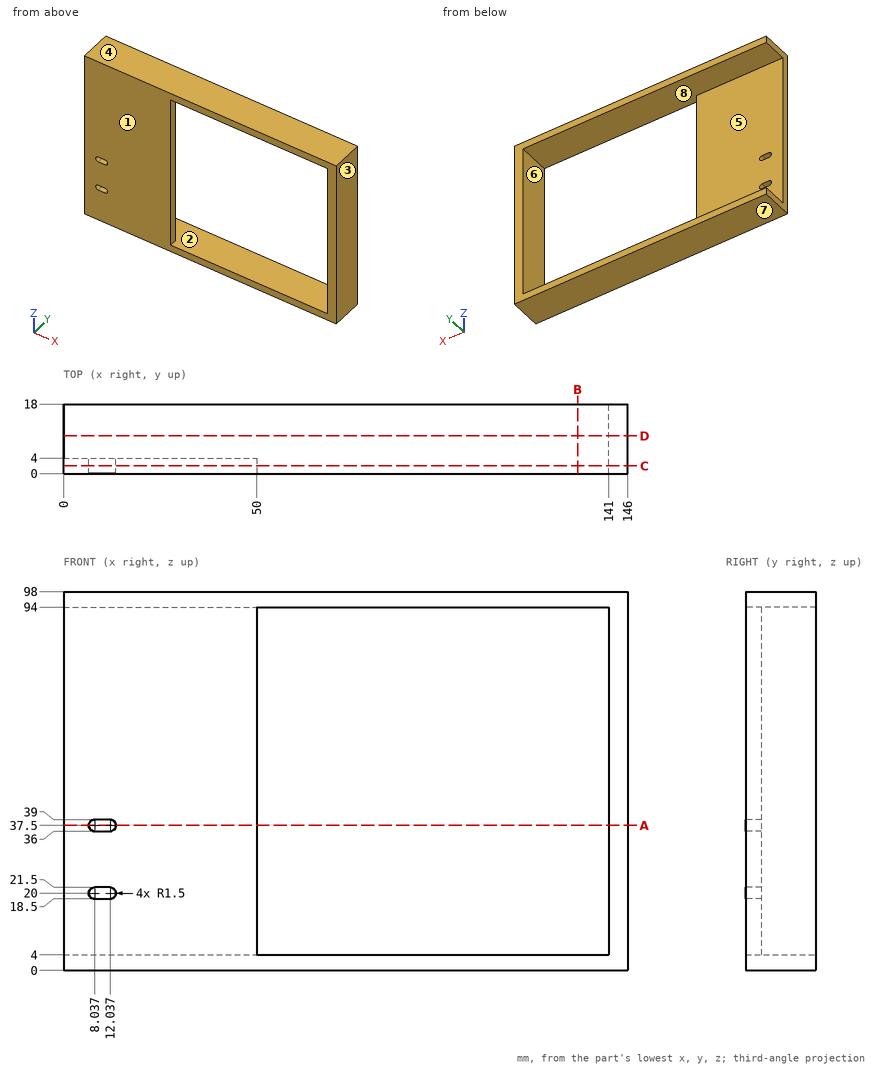
Study the drawing (mm; zero at the part's minimum x, y, z) and answer. A direction names the side the tool comes from. Round coordinates to 2 decimals unless told otherwise and drop trailing zeros. Write each loop counter-clockwise with the first axis right and the second up, starting at its lowest first coordinate (ties: lowest second). Pieces come first, ordered by that corner, then holes.
Q1. Find section A-A on z = 37.5. Determine the outline of the cut face in (x, y).
Values:
outline: (0, 0) - (6.54, 0) - (6.54, 4) - (0, 4) - close; (13.54, 0) - (50, 0) - (50, 4) - (13.54, 4) - close; (141, 0) - (146, 0) - (146, 18) - (141, 18) - close
Q2. Find section C-C on y = 2. Determine the outline of the cut face in (x, z).
Values:
outline: (0, 0) - (146, 0) - (146, 98) - (0, 98) - close; hole (8.04, 18.5) - (12.04, 18.5) arc R1.5 ccw to (12.04, 21.5) - (8.04, 21.5) arc R1.5 ccw to start; hole (8.04, 36) - (12.04, 36) arc R1.5 ccw to (12.04, 39) - (8.04, 39) arc R1.5 ccw to start; hole (50, 4) - (141, 4) - (141, 94) - (50, 94) - close
Q3. The mould has two halves that part along X. Classify the marked faces 1, 2 and 3: released by +X, released by -X, zero draft, split by the parting line, or undercut.
Values:
face 1: zero draft
face 2: undercut
face 3: released by +X
Q4. Flat-ended cylindrical pins translate along their axes: P1, Ø1, axis at x = 56.5, y = 11.5, coming from the -Z side; P2, Ø15, axis at x = 24.5, z = 55.5, coming from the +Y side; P3, Ø2, axis at y = 7.5, z = 68, coming from the -X side. Find the tip coordinate at first contact, or state that the pin passes through.
Values:
P1: stops at z = 0
P2: stops at y = 4
P3: stops at x = 141
Q5. Find section B-B on x = 133. Determine the outline of the cut face in (y, z).
Values:
outline: (0, 0) - (18, 0) - (18, 4) - (0, 4) - close; (0, 94) - (18, 94) - (18, 98) - (0, 98) - close
Q6. A tool of negligible diameter and unlimited length cuts with its end or side. For the marked faces 4, 5, 6, 7 and 8, from which of +Z, -Z, +X, -X, +Y, -Y can it reach the whole face along a straight path? Write none if from no direction.
Values:
face 4: +Z, +X, -X, +Y, -Y
face 5: -X, +Y
face 6: +Y, -Y
face 7: -Z, +X, -X, +Y, -Y
face 8: +Y
Q7. Straight lines are drawn through the part: line 1 (Z direction, x = 75, y = 6.75); line 2 (X direction, y = 3.5, z = 74); line 3 (Z direction, x = 7.5, y = 3.25). For each, find the intervals that lie inside material, in ascending order.
Values:
line 1: z = 0 to 4, 94 to 98
line 2: x = 0 to 50, 141 to 146
line 3: z = 0 to 18.6, 21.4 to 36.1, 38.9 to 98
Q8. Find section D-D on y = 9.75. Determine the outline of the cut face in (x, z), and give its area (3 significant figures).
Values:
outline: (0, 0) - (146, 0) - (146, 98) - (0, 98) - (0, 94) - (141, 94) - (141, 4) - (0, 4) - close
area: 1,620 mm2
